Geometry: final body of the model. Coordinates: model frame, mm. Face numbers are marked on the shaded views. A direction names the side the tool comes from. Give positions to 0.01 mm unless a question says otherwise; leave off trailing zeros. Loops run counter-clockwise (first coordinate to the right, second up) from the corner with the lowest first, then second, coordinate; pieces in that order, holes last.
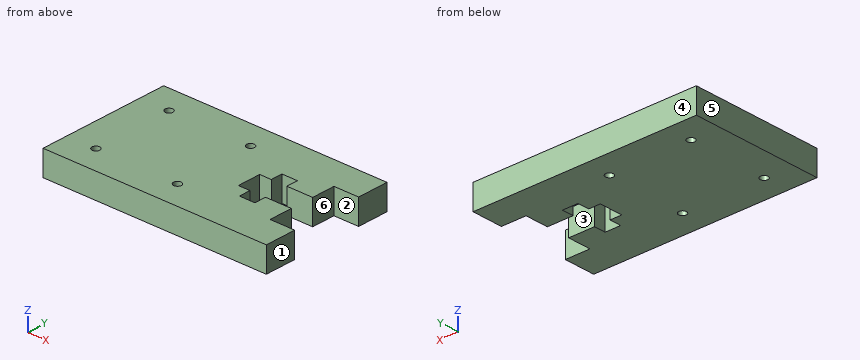
from build123d import *

# Parameters (mm, degrees)
F0_R     = 0.5
F1_DEPTH = 3.175


# Not quite as in the source:
# - a length typed as a fraction of an inch, garbled in the dataset ("3 / 203.2 mm" for 3/8 in), is restored


with BuildPart() as f1:
    # F0 (on Top) → F1 (new body)
    with BuildSketch(Plane.XY):
        Polygon((38.5022973402, 19.5465350598), (38.5022973402, 22.5465350598), (40.0022973402, 22.5465350598), (40.0022973402, 24.0465350598), (42.0022973402, 24.0465350598), (42.0022973402, 22.5465350598), (45.3272973402, 22.5465350598), (45.3272973402, 25.5465350598), (48.5022973402, 25.5465350598), (48.5022973402, 29.5465350598), (45.3272973402, 29.5465350598), (19.7522973402, 29.5465350598), (19.7522973402, 12.5465350598), (45.3272973402, 12.5465350598), (48.5022973402, 12.5465350598), (48.5022973402, 16.5465350598), (45.3272973402, 16.5465350598), (45.3272973402, 19.5465350598), (42.0022973402, 19.5465350598), (42.0022973402, 18.0465350598), (40.0022973402, 18.0465350598), (40.0022973402, 19.5465350598), align=None)
        with Locations((23.5022973402, 15.8965350598)):
            Circle(F0_R, mode=Mode.SUBTRACT)
        with Locations((34.0022973402, 15.8965350598)):
            Circle(F0_R, mode=Mode.SUBTRACT)
        with Locations((23.5022973402, 26.1965350598)):
            Circle(F0_R, mode=Mode.SUBTRACT)
        with Locations((34.0022973402, 26.1965350598)):
            Circle(F0_R, mode=Mode.SUBTRACT)
    extrude(amount=F1_DEPTH)


solid = f1.part
Item 1: Ray query, probe 1 along X at (y, z) = (26.5, 2); probe 2 along X at (y, z) = (23, 0.9); probe 3 along Y at (x, z) = (41.5, 1.65). Return the intervals inside material, ascending.
Values follow:
probe 1: x = 19.75 to 23.1, 23.9 to 33.6, 34.4 to 48.5
probe 2: x = 19.75 to 40, 42 to 45.33
probe 3: y = 12.55 to 18.05, 24.05 to 29.55
Item 2: Section query B-B on y = 19. Return loops of the section in (x, z) (3 decimals).
Values follow:
outline: (19.752, 0) - (40.002, 0) - (40.002, 3.175) - (19.752, 3.175) - close; (42.002, 0) - (45.327, 0) - (45.327, 3.175) - (42.002, 3.175) - close
Item 3: Section query D-D on y = 25. Return loops of the section in (x, z) (3 decimals), plus the area to 3 significant figures.
Values follow:
outline: (19.752, 0) - (45.327, 0) - (45.327, 3.175) - (19.752, 3.175) - close
area: 81.2 mm2
Item 4: Draft query along Y for the marked faces 1, 2, 3 and 4. Return one class per face: +Y half, -Y half, draft (parallel to the pull), parting line (faces both ways), or undercut.
Values follow:
face 1: draft
face 2: undercut
face 3: undercut
face 4: +Y half
Item 5: Section query A-A on x = 40.75. Return loops of the section in (y, z) (3 decimals), plus the area to 3 significant figures.
Values follow:
outline: (12.547, 0) - (18.047, 0) - (18.047, 3.175) - (12.547, 3.175) - close; (24.047, 0) - (29.547, 0) - (29.547, 3.175) - (24.047, 3.175) - close
area: 34.9 mm2
Item 6: Pin query (flat end, axial travel): pin 1 (0.8 mm diameter, centred on y = 19, z = 1.5, fed in from +X); pin 2 (1.5 mm diameter, centred on y = 21, z = 2, fed in from +X). Return the tip coordinate at first contact, or that it passes through.
Values follow:
pin 1: stops at x = 45.33
pin 2: stops at x = 38.5
Item 7: Set-up query: the marked faces 5 and 6. Return all of +Z, -Z, +X, -X, +Y, -Y with unobstructed straight access to the full face (end or side cutting, diameter ignored); none if empty.
Values follow:
face 5: +Z, -Z, -X, +Y, -Y
face 6: +Z, -Z, +X
Item 8: Section query C-C on z = 2. Return loops of the section in (x, y).
Values follow:
outline: (19.75, 12.55) - (48.5, 12.55) - (48.5, 16.55) - (45.33, 16.55) - (45.33, 19.55) - (42, 19.55) - (42, 18.05) - (40, 18.05) - (40, 19.55) - (38.5, 19.55) - (38.5, 22.55) - (40, 22.55) - (40, 24.05) - (42, 24.05) - (42, 22.55) - (45.33, 22.55) - (45.33, 25.55) - (48.5, 25.55) - (48.5, 29.55) - (19.75, 29.55) - close; hole circle Ø1 at (23.5, 15.9); hole circle Ø1 at (23.5, 26.2); hole circle Ø1 at (34, 15.9); hole circle Ø1 at (34, 26.2)
